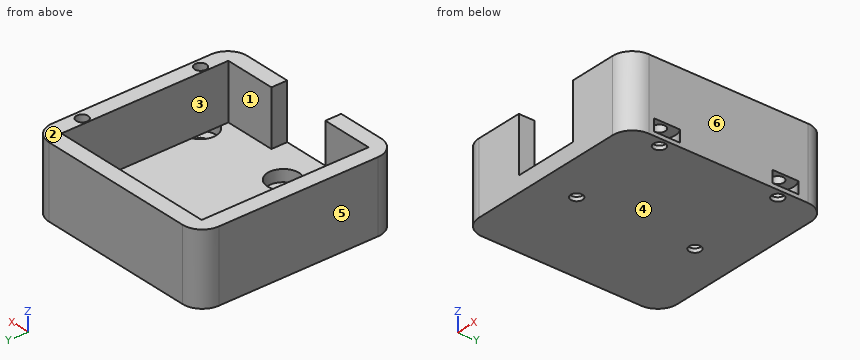
```python
from build123d import *

# Parameters (mm, degrees)
ESQUISSE1_W             = 50.3
ESQUISSE1_H             = 50.3
BOSS_EXTRU_1_DEPTH      = 4
BOSS_EXTRU_2_DEPTH      = 14
ESQUISSE3_R             = 1.5
ENL_V_MAT_EXTRU_1_DEPTH = 74.376971864
CONG_2_R                = 5
ESQUISSE4_R             = 4
ENL_V_MAT_EXTRU_2_DEPTH = 3
CONG_6_R                = 5


with BuildPart() as part:
    # Esquisse1 → Boss.-Extru.1 (new body)
    with BuildSketch(Plane.XY):
        with Locations((25.15, 25.15)):
            Rectangle(ESQUISSE1_W, ESQUISSE1_H)
    extrude(amount=BOSS_EXTRU_1_DEPTH)

    # Esquisse2 → Boss.-Extru.2 (add)
    with BuildSketch(Plane.XY.offset(4)):
        Polygon((4, 46.3), (46.3, 46.3), (46.3, 4), (33.3, 4), (33.3, 0), (50.3, 0), (50.3, 50.3), (0, 50.3), (0, 0), (17, 0), (17, 4), (4, 4), align=None)
    extrude(amount=BOSS_EXTRU_2_DEPTH)

    # Esquisse3 → Enlèv. mat.-Extru.1 (cut, through all)
    with BuildSketch(Plane(origin=(0, 0, 0), x_dir=(-1, 0, 0), z_dir=(0, 0, -1))):
        with Locations((-23.024217253, 39.6)):
            Circle(ESQUISSE3_R)
        with Locations((-48.024217253, 39.6)):
            Circle(ESQUISSE3_R)
        with Locations((-48.024217253, 9.6)):
            Circle(ESQUISSE3_R)
        with Locations((-23.024217253, 9.6)):
            Circle(ESQUISSE3_R)
    extrude(amount=-ENL_V_MAT_EXTRU_1_DEPTH, mode=Mode.SUBTRACT)

    # Congé2
    cong_2_edges = [part.edges().sort_by_distance(p)[0] for p in [
        (0, 50.3, 9),
    ]]
    fillet(cong_2_edges, radius=CONG_2_R)

    # Esquisse4 → Enlèv. mat.-Extru.2 (cut)
    with BuildSketch(Plane.XY.offset(4)):
        with Locations((23.024217253, 39.6)):
            Circle(ESQUISSE4_R)
        with Locations((23.024217253, 9.6)):
            Circle(ESQUISSE4_R)
        with Locations((48.024217253, 39.6)):
            Circle(ESQUISSE4_R)
        with Locations((48.024217253, 9.6)):
            Circle(ESQUISSE4_R)
    extrude(amount=-ENL_V_MAT_EXTRU_2_DEPTH, mode=Mode.SUBTRACT)

    # Congé6
    cong_6_edges = [part.edges().sort_by_distance(p)[0] for p in [
        (50.3, 50.3, 9),
        (50.3, 0, 9),
        (0, 0, 9),
    ]]
    fillet(cong_6_edges, radius=CONG_6_R)


solid = part.part
```
Read the model definition and answer for the solid it produces. Units are mm, in the model's axes. Face numbers are marked on the shaded views. A direction names the side the tool comes from. Coordinates: 2 decimals unless noted, no trailing zeros. Write each loop counter-clockwise with the first axis right and the second up, starting at its lowest first coordinate (ties: lowest second). Pieces come first, ordered by that corner, then holes. Notation, with made-up numbers: (1, 28.5) -> (36, 28.5) arc R18 cw to (36, 50.5) -> close; hole circle Ø8 at (31, 36). An arc over 180 degrees is marked (long way). Return JSON: item names as keys, results as strings.
1. A cutting plane is placed at C-C (x = 11). Determine the outline of the cut face in (y, z).
Found:
{"outline": "(0, 0) -> (50.3, 0) -> (50.3, 18) -> (46.3, 18) -> (46.3, 4) -> (4, 4) -> (4, 18) -> (0, 18) -> close"}
2. A cutting plane is placed at B-B (z = 7.5). Determine the outline of the cut face in (x, y).
Found:
{"outline": "(0, 5) arc R5 ccw to (5, 0) -> (17, 0) -> (17, 4) -> (4, 4) -> (4, 46.3) -> (46.3, 46.3) -> (46.3, 4) -> (33.3, 4) -> (33.3, 0) -> (45.3, 0) arc R5 ccw to (50.3, 5) -> (50.3, 45.3) arc R5 ccw to (45.3, 50.3) -> (5, 50.3) arc R5 ccw to (0, 45.3) -> close; hole circle Ø3 at (48.02, 9.6); hole circle Ø3 at (48.02, 39.6)"}
3. Determine the mould class of the marked faces 3, 4, 5 and 6 for opening direction X: pulls with the +X half, pulls with the -X half, needs draft (parallel to the pull), parting line crosses it, or undercut.
Found:
{"face 3": "undercut", "face 4": "needs draft", "face 5": "pulls with the -X half", "face 6": "pulls with the +X half"}
4. Find the intervals of material crossed by line 1 along Y through (x, z) = (12, 12.5); line 2 along X through (y, z) = (39, 5.25), in increasing order. Write a range as from..to.
Found:
{"line 1": "0..4, 46.3..50.3", "line 2": "0..4, 46.3..46.65, 49.4..50.3"}
5. A cutting plane is placed at A-A (y = 39.6). Determine the outline of the cut face in (x, z), and give its area (3 significant figures).
Found:
{"outline": "(0, 0) -> (21.52, 0) -> (21.52, 1) -> (19.02, 1) -> (19.02, 4) -> (4, 4) -> (4, 18) -> (0, 18) -> close; (24.52, 0) -> (46.52, 0) -> (46.52, 1) -> (44.02, 1) -> (44.02, 4) -> (27.02, 4) -> (27.02, 1) -> (24.52, 1) -> close; (46.3, 4) -> (46.52, 4) -> (46.52, 18) -> (46.3, 18) -> close; (49.52, 0) -> (50.3, 0) -> (50.3, 1) -> (49.52, 1) -> close; (49.52, 4) -> (50.3, 4) -> (50.3, 18) -> (49.52, 18) -> close", "area": "222 mm2"}
6. Each of these flat-tipped pins is pushed along its axis until it touches: P1, Ø4, axis at x = 24.5, y = 9.5, coming from the +Z side; P2, Ø3, axis at x = 21, z = 9.5, coming from the -Y side; P3, Ø4, axis at x = 41.5, y = 26.5, coming from the +Z side; P4, Ø2.5, axis at x = 48.02, y = 9.6, coming from the -Z side. Where does it stop, or does it pass through?
Found:
{"P1": "z = 1", "P2": "y = 46.3", "P3": "z = 4", "P4": "through"}
7. A tool of negligible diameter and unlimited length cuts with its end or side. For the marked faces 1 and 2, from which of +Z, -Z, +X, -X, +Y, -Y can it reach the whole face along a straight path? Write none if from no direction.
Found:
{"face 1": "+Z", "face 2": "+Z, +X, -X, +Y, -Y"}
